Autodesk Inventor part; units mm, degrees
ref_plane "YZ Plane" through (0, 0, 0) normal (1, 0, 0) x (0, 1, 0)
ref_plane "XZ Plane" through (0, 0, 0) normal (0, 1, 0) x (-1, 0, 0)
ref_plane "XY Plane" through (0, 0, 0) normal (0, 0, 1) x (1, 0, 0)
sketch "スケッチ1" plane through (0, 0, 0) normal (0, 0, 1) x (1, 0, 0)
  line L0 (-5.5, -10) -> (5.5, -10)
  line L1 (5.5, -10) -> (5.5, 10)
  line L2 (5.5, 10) -> (-5.5, 10)
  line L3 (-5.5, 10) -> (-5.5, -10)
  line L4 (-5.5, -10) -> (5.5, 10) construction
  line L5 (5.5, -10) -> (-5.5, 10) construction
  point P0 (0, 0)
  dimension "d0" = 11
  dimension "d1" = 20
extrude "プレート1" add sketch "スケッチ1" along normal blind 3
sketch "スケッチ2" plane through (8.5, -10, -3) normal (1, 0, 0) x (0, 1, 0)
  line L0 (20, 0) -> (0, 0)
  line L1 (0, 0) -> (0, -15)
  line L2 (0, -15) -> (20, -15)
  line L3 (20, -15) -> (20, 0)
edge flange "フランジ1" height 21 angle 90 thickness 3 bend radius 3 thickness toward (1, 0, 0) relief tear relief width 3 relief depth 1.5 edges at (5.5, 0, 0) wall of the first edge with corners at (8.5, 10, -3) (8.5, -10, -3) (8.5, -10, -18) (8.5, 10, -18)
bend "曲げ1"
corner "コーナー1"
sketch "スケッチ3" plane through (0, 0, 3) normal (0, 0, 1) x (1, 0, 0)
  line L0 (-5.5, -10) -> (-5.5, 10)
  line L1 (5.5, -10) -> (-5.5, -10)
  line L2 (5.5, 10) -> (5.5, -10)
  line L3 (-5.5, 10) -> (5.5, 10)
  point P0 (-1.5, 0)
  dimension "d29" = 4
hole "穴1" at (-1.5, 0, 3) direction (0, 0, -1) diameter 3.242 end through all
sketch "スケッチ4" plane through (11.5, -10, -18) normal (1, 0, 0) x (0, 0, -1)
  line L0 (-15, 20) -> (-15, 0)
  line L1 (0, 0) -> (-15, 0)
  line L2 (0, 20) -> (0, 0)
  line L3 (-15, 20) -> (0, 20)
  point P0 (-18, 10)
  point P1 (-7.5, 10)
  dimension "d20" = 7.5
hole "穴2" at (11.5, 0, -10.5) direction (-1, 0, 0) diameter 6.2 end through all
fillet "フィレット1" radius 2 4 edges at (-5.5, 10, 1.5) (-5.5, -10, 1.5) (10, -10, -18) (10, 10, -18)
equation "\"d2\" = Thickness"
equation "\"d3\" = BendReliefWidth"
equation "\"d4\" = BendReliefDepth"
equation "\"d5\" = MinimumRemnant"
equation "\"d6\" = TransitionRadius"
equation "\"d9\" = BendRadius"
equation "\"d10\" = CornerReliefSize"
equation "\"d11\" = GapSize"
equation "\"d12\" = JacobiRadiusSize"
equation "\"BendRadius\" = Thickness"
equation "\"BendReliefWidth\" = Thickness"
equation "\"BendReliefDepth\" = 0.5 * Thickness"
equation "\"CornerReliefSize\" = 4 * Thickness"
equation "\"MinimumRemnant\" = 2 * Thickness"
equation "\"TransitionRadius\" = BendRadius"
equation "\"JacobiRadiusSize\" = BendRadius"
equation "\"GapSize\" = Thickness"
properties part number "Belt_Tenshon_Meviy"
Could you check a few things on this model? Use its own coordinates, in mm. A direction names the side the tool comes from. Round coordinates to 2 decimals unless told otherwise and drop trailing zeros. Loops run counter-clockwise (first coordinate to the right, second up) from the corner with the lowest first, then second, coordinate; pieces in that order, holes last. Notation, with made-up numbers: (46, 78.5) -> (98, 78.5) arc R23 ccw to (98, 98.5) -> close; hole circle Ø5 at (-9, 29). An arc over 180 degrees is marked (long way). Use CSV: the item, a comma, the result in double quotes.
(1) If we mould it in two halves opening along Z, with no side actions, what happens to faces 3 (the cylindrical face through (10, -0.1, -7.4)), 4 (the cylindrical face through (9.789, -0.14, 1.196)), 5 (the flat face through (9, -10, -3))? For each: +Z half, -Z half, draft (parallel to the pull), parting line (faces both ways), or undercut.
Return value:
face 3,"undercut"
face 4,"+Z half"
face 5,"draft"
(2) Suppose I cut it at C-C on x = 9. Write out the boundary of the cut face in (y, z), plus the area to 3 significant figures.
Return value:
outline,"(-10, -16) arc R2 ccw to (-8, -18) -> (8, -18) arc R2 ccw to (10, -16) -> (10, 1.87) -> (-10, 1.87) -> close; hole circle Ø6.2 at (0, -10.5)"
area,"366 mm²"
(3) Will these pins go through, and if not, where does the flat tip stop? pin 1 Ø9 at (x, y) = (2.5, -2) entering from -Z; pin 2 Ø10 at (y, z) = (-7.5, -6.5) entering from -X; pin 3 Ø10 at (x, y) = (3, 2) entering from -Z.
Return value:
pin 1,"stops at z = -0.4"
pin 2,"stops at x = 8.1"
pin 3,"stops at z = -1.34"
(4) Suppose I cut it at B-B on z = -10.5. Write out the boundary of the cut face in (x, y).
Return value:
outline,"(8.5, -10) -> (11.5, -10) -> (11.5, -3.1) -> (8.5, -3.1) -> close; (8.5, 3.1) -> (11.5, 3.1) -> (11.5, 10) -> (8.5, 10) -> close"
(5) If I drill on probe 1 along Y at (x, z) = (9.3, -10.5); probe 2 along Y at (x, z) = (-1.5, 1.45); probe 3 along X at (y, z) = (-9, -14.5), over which ranges is the centre line in solid material (lowest first)? Write a range as [from, to].
Return value:
probe 1,"y = [-10, -3.1], [3.1, 10]"
probe 2,"y = [-10, -1.62], [1.62, 10]"
probe 3,"x = [8.5, 11.5]"
(6) Suppose I cut it at D-D on y = -3.5. Write out the boundary of the cut face in (x, z).
Return value:
outline,"(-5.5, 0) -> (5.5, 0) arc R3 cw to (8.5, -3) -> (8.5, -18) -> (11.5, -18) -> (11.5, -3) arc R6 ccw to (5.5, 3) -> (-5.5, 3) -> close"
(7) Suppose I cut it at A-A on y = 0. Write out the boundary of the cut face in (x, z), plus the area to 3 significant figures.
Return value:
outline,"(-5.5, 0) -> (-3.12, 0) -> (-3.12, 3) -> (-5.5, 3) -> close; (0.12, 0) -> (5.5, 0) arc R3 cw to (8.5, -3) -> (8.5, -7.4) -> (11.5, -7.4) -> (11.5, -3) arc R6 ccw to (5.5, 3) -> (0.12, 3) -> close; (8.5, -18) -> (11.5, -18) -> (11.5, -13.6) -> (8.5, -13.6) -> close"
area,"70.9 mm²"
(8) For faces 1 (the flat face through (1, 0, 0)), 2 (the cylindrical face through (-4.93, -9.4, 1.52)), which set-ups out of +Z, -Z, +X, -X, +Y, -Y let a thin tool reach every point of the face, with its end or its side?
Return value:
face 1,"-Z, -X, +Y, -Y"
face 2,"+Z, -Z, -X, -Y"
